```python
from build123d import *

# Parameters (mm, degrees)
SKETCH7_R               = 2.9999999999999982
SKETCH7_R_2             = 1.0000000000000018
SKETCH7_R_3             = 3.0000000000000018
SKETCH7_R_4             = 0.9999999999999983
BOSS_EXTRUDE1_DEPTH     = 2
SKETCH9_R               = 0.9999999999999983
BOSS_EXTRUDE2_DEPTH     = 4
CUT_EXTRUDE3_DEPTH      = 68.5610601855979
CUT_EXTRUDE3_DEPTH_BACK = 68.5610601855979
CHAMFER1_SIZE           = 2
FILLET10_R              = 0.75


with BuildPart() as part:
    # Sketch7 → Boss-Extrude1 (new, symmetric)
    # profile 1 of 3: a face of its own
    with BuildSketch(Plane.XY):
        with BuildLine():
            Line((11.893863235859584, 53.137939029439345), (15.445357626885196, 44.86830254465274))
            ThreePointArc((15.445357626885198, 44.86830254465274), (16.642699652600193, 45.857903547949306), (18.174468795559314, 46.11601469638566))
            Line((18.174468795559314, 46.11601469638567), (15.526434240422798, 52.28194958437761))
            Line((15.526434240422798, 52.28194958437761), (39.886948210676515, 72.89692053805315))
            ThreePointArc((39.88694821067651, 72.89692053805315), (38.98584570958542, 74.39162614577609), (39.06921198001558, 76.13495073866909))
            Line((39.06921198001558, 76.13495073866909), (11.893863235859584, 53.137939029439345))
        make_face()
    # profile 2 of 3: a face of its own
    with BuildSketch(Plane.XY):
        with Locations((17.890076901850104, 43.12952490889392)):
            Circle(SKETCH7_R)
        with Locations((17.890076901850104, 43.12952490889392)):
            Circle(SKETCH7_R_2, mode=Mode.SUBTRACT)
    # profile 3 of 3: a face of its own
    with BuildSketch(Plane.XY):
        with Locations((41.8945256681437, 75.12618785093188)):
            Circle(SKETCH7_R_3)
        with Locations((41.8945256681437, 75.12618785093188)):
            Circle(SKETCH7_R_4, mode=Mode.SUBTRACT)
    extrude(amount=BOSS_EXTRUDE1_DEPTH, both=True)

    # Sketch9 → Boss-Extrude2 (add, symmetric)
    with BuildSketch(Plane.XY):
        with BuildLine():
            Line((17.43729995500307, 47.832508562943936), (18.174468795559275, 46.11601469638567))
            ThreePointArc((18.174468795559275, 46.11601469638567), (19.137454151100034, 40.40114626983855), (15.4453576268852, 44.86830254465274))
            Line((15.4453576268852, 44.86830254465274), (14.680754460074215, 46.64867709926875))
            Line((14.680754460074215, 46.64867709926875), (17.43729995500307, 47.832508562943936))
        make_face()
        with Locations((17.890076901850104, 43.12952490889392)):
            Circle(SKETCH9_R, mode=Mode.SUBTRACT)
    extrude(amount=BOSS_EXTRUDE2_DEPTH, both=True)

    # Sketch10 → Cut-Extrude3 (cut, two sides: drawn at the far end of the back side and taken through both)
    with BuildSketch(Plane(origin=(32.06546623724915, 13.770898357710635, 0), x_dir=(0, 0, -1), z_dir=(0.9188484983096216, 0.39461048789173536, 0)).offset(-CUT_EXTRUDE3_DEPTH_BACK)):
        Polygon((1.9999999999999996, 27.385841036947262), (-1.9999999999999991, 27.385841036947262), (-1.9999999999999996, 35.88584103694727), (2.0000000000000004, 35.88584103694727), align=None)
    extrude(amount=CUT_EXTRUDE3_DEPTH + CUT_EXTRUDE3_DEPTH_BACK, mode=Mode.SUBTRACT)

    # Chamfer1
    chamfer1_edges = [part.edges().sort_by_distance(p)[0] for p in [
        (16.05902720753864, 47.24059283110634, -4),
        (16.05902720753864, 47.24059283110634, 4),
    ]]
    chamfer(chamfer1_edges, length=CHAMFER1_SIZE - 0.0001)  # a hair under: the kernel refuses the full size

    # Fillet10
    fillet10_edges = [part.edges().sort_by_distance(p)[0] for p in [
        (16.526264249789705, 46.15263377324982, -2.0000000000000004),
        (16.526264249789676, 46.15263377324982, 1.9999999999999996),
    ]]
    fillet(fillet10_edges, radius=FILLET10_R)


solid = part.part
```
Model file for the job. Use its own axes, mm. A direction names the side the tool comes from. Coordinates: 2 decimals unless noted, no trailing zeros. Loops run counter-clockwise (first coordinate to the right, second up) from the corner with the lowest first, then second, coordinate; pieces in that order, holes last. Notation, with made-up numbers: (-18.5, -4.75) - (13.5, -4.75) arc R13 cw to (13.5, 7.25) - close; hole circle Ø4 at (-32.75, 2.25). An arc over 180 degrees is marked (long way). Write item = value, one per line. Start each with the question number.
Item 1: Saw through at B-B, the plane z = 0.5. List the corners of the cut face in (x, y), then the cut area to 3 significant figures.
Item 2: Saw through at C-C, the plane y = 49.5. List the corners of the cut face in (x, z), then the cut area to 3 significant figures.
Item 3: Saw through at A-A, the plane x = 41.5. List the corners of the cut face in (y, z).
Item 4: 3-axis set-ups, long thin cutter, end or side, ignore diameter. For faces 4 (the face through (16.832, 49.242, 0.054)), 5 (the face through (16.507, 46.144, 0.017)), 6 (the face through (16.493, 46.324, 3.014)): which of +Z, -Z, +X, -X, +Y, -Y reach the whole face in a straight line?
Item 5: Saw through at D-D, the plane x = 32. List the corners of the cut face in (y, z), then the cut area to 3 significant figures.
Item 6: Wall check: probe 1 along X at (y, z) = (42.5, -3); probe 2 along X at (y, z) = (72.5, 0); probe 3 along Y at (x, z) = (22, 1.5). Give the ranges that are in metal, low to high. Write a range as [from, to].
Item 7: Pull direction X, two halves, no side cores. Call faces 1 (the face through (17.76, 44.12, -3.01)), 2 (the face through (25.672, 64.797, 0.028)), 3 (the face through (18.4, 41.8, -2)): +X half, -X half, draft (parallel to the pull), parting line (faces both ways), or undercut.
Item 8: Drop flat-ended pins along their axis: pin 1 Ø15.5 at (x, y) = (27, 65.5) entering from +Z; pin 2 Ø2.5 at (x, y) = (41.89, 75.13) entering from -Z; pin 3 Ø1.6 at (x, y) = (41.89, 75.13) entering from +Z; pin 4 Ø1.5 at (y, z) = (44.5, 1.5) entering from +X. Give the stop position or say it passes through.
Answers:
q1.outline = (11.89, 53.14) - (15.15, 45.56) - (17.9, 46.74) - (15.53, 52.28) - (39.89, 72.9) arc R3 ccw (long way) to (39.07, 76.13) - close; hole circle Ø2 at (41.89, 75.13)
q1.area = 147 mm2
q2.outline = (13.46, -2) - (16.72, -2) - (16.72, 2) - (13.46, 2) - close
q2.area = 13.1 mm2
q3.outline = (72.15, -2) - (74.21, -2) - (74.21, 2) - (72.15, 2) - close; (76.05, -2) - (78.1, -2) - (78.1, 2) - (76.05, 2) - close
q4.face_4 = +Z, -Z, +X
q4.face_5 = +X, -Y
q4.face_6 = +Z, -X, +Y
q5.outline = (66.22, -2) - (70.15, -2) - (70.15, 2) - (66.22, 2) - close
q5.area = 15.7 mm2
q6.probe_1 = [14.96, 17.11], [18.67, 20.82]
q6.probe_2 = [34.77, 39.42], [40.44, 43.34]
q6.probe_3 = [57.76, 61.69]
q7.face_1 = undercut
q7.face_2 = -X half
q7.face_3 = draft
q8.pin_1 = 2
q8.pin_2 = -2
q8.pin_3 = through
q8.pin_4 = 20.78
